Geometry check sheet. Reference: the model listing, model coordinates, mm. A direction names the side the tool comes from. Give positions to 0.01 mm unless a question says otherwise; leave off trailing zeros. Write each loop counter-clockwise with the first axis right and the second up, starting at its lowest first coordinate (ties: lowest second). Pieces come first, ordered by that corner, then holes. Notation, with made-up numbers: (-10, 25) -> (10, 25) arc R30 ccw to (10, 57) -> close; hole circle Ø5 at (84, 77.5). An arc over 180 degrees is marked (long way). Write item = value, one per line. Start each with the question number.
1. Thickness scan on line 1 along Y through (x, z) = (0, 3.25); line 2 along Y through (x, z) = (0, 10.1); line 3 along Z through (x, y) = (3.3, 0). Record the ranges inside material, lowest first.
2. Mould release check, pull along Y, two halves, no side actions. Record for faces 1 (the cylindrical face through (0.098, -0.756, 2.465)), 2 (the flat face through (0, 1, 14)), 3 (the cylindrical face through (-0.845, -3.807, 6.909)): pulls with the +Y half, pulls with the -Y half, needs draft (parallel to the pull), parting line crosses it, or undercut.
3. Cross-section at B-B, the plane y = 0. Record the cut outline in (x, z), plus the area to 3 significant figures.
4. Cross-section at A-A, the plane x = 0. Record the cut outline in (y, z), plus the area to 3 significant figures.
5. Cross-section at C-C, the plane z = 10.75. Record the cut outline in (x, y), plus the area to 3 significant figures.
6. Depth check by flat-ended pin: P1, Ø2, axis at x = 0, y = 1.5, coming from the -Z side; P2, Ø1, axis at y = 1, z = 8, coming from the -X side; P3, Ø0.8, axis at x = 0, y = 0, coming from the +Z side; P4, Ø1.1, axis at y = -0.5, z = 8, coming from the +X side. Enter the tip coordinate at first touch or a pass-through.
7. Set-up check for faces 4 (the cylindrical face through (-3.173, -0.287, 6.604)), 5 (the cylindrical face through (3.173, -0.287, 6.604)), 6 (the cylindrical face through (0.163, 0.768, 2.465)): record each of +Z, -Z, +X, -X, +Y, -Y from which the full face is reachable in a straight line by a thin tool's end or side.
```python
from build123d import *

# Parameters (mm, degrees)
SKETCH1_R           = 3.9
BOSS_EXTRUDE1_DEPTH = 14
FILLET1_R           = 0.5
SKETCH2_R           = 0.75
CUT_EXTRUDE2_DEPTH  = 5
SKETCH3_R           = 0.75
CUT_EXTRUDE3_DEPTH  = 5
SKETCH4_R           = 0.75
CUT_EXTRUDE4_DEPTH  = 1
SKETCH5_W           = 0.434986795
SKETCH5_H           = 2.227981147
CUT_EXTRUDE5_DEPTH  = 2.8


with BuildPart() as part:
    # Sketch1 → Boss-Extrude1 (new body)
    with BuildSketch(Plane.XY):
        Circle(SKETCH1_R)
    extrude(amount=BOSS_EXTRUDE1_DEPTH)

    # Fillet1
    fillet1_edges = [part.edges().sort_by_distance(p)[0] for p in [
        (-3.9, 0, 0),
        (-3.9, 0, 14),
    ]]
    fillet(fillet1_edges, radius=FILLET1_R)

    # Sketch2 → Cut-Extrude2 (cut)
    with BuildSketch(Plane.XY.offset(14)):
        Circle(SKETCH2_R)
    extrude(amount=-CUT_EXTRUDE2_DEPTH, mode=Mode.SUBTRACT)

    # Sketch3 → Cut-Extrude3 (cut)
    with BuildSketch(Plane(origin=(0, 0, 0), x_dir=(-1, 0, 0), z_dir=(0, 0, -1))):
        with Locations((0, 1.5)):
            Circle(SKETCH3_R)
        with Locations((0, -1.5)):
            Circle(SKETCH3_R)
    extrude(amount=-CUT_EXTRUDE3_DEPTH, mode=Mode.SUBTRACT)

    # Sketch4 → Cut-Extrude4 (cut, symmetric)
    with BuildSketch(Plane(origin=(-3.8, 0, 0), x_dir=(0, 0, -1), z_dir=(1, 0, 0))):
        with Locations((-7.297217633, 0)):
            Circle(SKETCH4_R)
    cut_extrude4 = extrude(amount=CUT_EXTRUDE4_DEPTH, both=True, mode=Mode.SUBTRACT)

    # Sketch5 → Cut-Extrude5 (cut)
    with BuildSketch(Plane.XY.offset(6)):
        with Locations((-3.774117143, 0.125124808)):
            Rectangle(SKETCH5_W, SKETCH5_H)
    cut_extrude5 = extrude(amount=CUT_EXTRUDE5_DEPTH, mode=Mode.SUBTRACT)

    # Mirror1: Cut-Extrude4, Cut-Extrude5 across plane
    add(cut_extrude4.mirror(Plane(origin=(0, 0, 0), x_dir=(0, 0, 1), z_dir=(1, 0, 0))), mode=Mode.SUBTRACT)
    add(cut_extrude5.mirror(Plane(origin=(0, 0, 0), x_dir=(0, 0, 1), z_dir=(1, 0, 0))), mode=Mode.SUBTRACT)


solid = part.part
```
Answers:
q1.line_1 = -3.9 to -2.25, -0.75 to 0.75, 2.25 to 3.9
q1.line_2 = -3.9 to -0.75, 0.75 to 3.9
q1.line_3 = 0 to 6.55, 8.05 to 14
q2.face_1 = undercut
q2.face_2 = needs draft
q2.face_3 = parting line crosses it
q3.outline = (-3.9, 0.5) arc R0.5 ccw to (-3.4, 0) -> (3.4, 0) arc R0.5 ccw to (3.9, 0.5) -> (3.9, 6) -> (3.56, 6) -> (3.56, 6.55) -> (2.8, 6.55) -> (2.8, 8.05) -> (3.56, 8.05) -> (3.56, 8.8) -> (3.9, 8.8) -> (3.9, 13.5) arc R0.5 ccw to (3.4, 14) -> (0.75, 14) -> (0.75, 9) -> (-0.75, 9) -> (-0.75, 14) -> (-3.4, 14) arc R0.5 ccw to (-3.9, 13.5) -> (-3.9, 8.8) -> (-3.56, 8.8) -> (-3.56, 8.05) -> (-2.8, 8.05) -> (-2.8, 6.55) -> (-3.56, 6.55) -> (-3.56, 6) -> (-3.9, 6) -> close
q3.area = 97.3 mm^2
q4.outline = (-3.9, 0.5) arc R0.5 ccw to (-3.4, 0) -> (-2.25, 0) -> (-2.25, 5) -> (-0.75, 5) -> (-0.75, 0) -> (0.75, 0) -> (0.75, 5) -> (2.25, 5) -> (2.25, 0) -> (3.4, 0) arc R0.5 ccw to (3.9, 0.5) -> (3.9, 13.5) arc R0.5 ccw to (3.4, 14) -> (0.75, 14) -> (0.75, 9) -> (-0.75, 9) -> (-0.75, 14) -> (-3.4, 14) arc R0.5 ccw to (-3.9, 13.5) -> close
q4.area = 86.5 mm^2
q5.outline = circle Ø7.8 at (0, 0); hole circle Ø1.5 at (0, 0)
q5.area = 46.0 mm^2
q6.P1 = 0
q6.P2 = -3.7
q6.P3 = 9
q6.P4 = 3.77
q7.face_4 = -X
q7.face_5 = +X
q7.face_6 = -Z
